```python
from build123d import *

# Parameters (mm, degrees)
BOSS_EXTRUDE1_DEPTH     = 40
SKETCH2_R               = 12.5
CUT_EXTRUDE1_DEPTH      = 4.4775
FILLET1_R               = 10
CUT_EXTRUDE2_DEPTH      = 131.2
CUT_EXTRUDE2_DEPTH_BACK = 14.2
SKETCH4_R               = 2.5
SKETCH6_W               = 68
SKETCH6_H               = 90
BOSS_EXTRUDE4_DEPTH     = 10
FILLET2_R               = 10
FILLET3_R               = 5
FILLET4_R               = 4
CUT_EXTRUDE3_START      = -2.2025
SKETCH7_R               = 3.9
CUT_EXTRUDE3_DEPTH      = 0.85
SKETCH8_R               = 3.25
CUT_EXTRUDE4_DEPTH      = 10
SKETCH9_R               = 4.025
CUT_EXTRUDE5_DEPTH      = 12
SKETCH10_W              = 20.05
SKETCH10_H              = 20.05
CUT_EXTRUDE6_DEPTH      = 4
CUT_EXTRUDE7_DEPTH      = 6
CUT_EXTRUDE9_DEPTH      = 2.5
CUT_EXTRUDE10_REACH     = 138.104
CUT_EXTRUDE10_START     = -2.5
SKETCH15_R              = 1.5
FILLET5_R               = 3


with BuildPart() as part:
    # Sketch1 → Boss-Extrude1 (new body)
    with BuildSketch(Plane.XY):
        Polygon((10, 0), (10, 43), (104, 43), (104, 0), (114, 0), (114, 53), (0, 53), (0, 0), align=None)
    extrude(amount=-BOSS_EXTRUDE1_DEPTH)

    # Sketch2 → Cut-Extrude1 (cut)
    with BuildSketch(Plane(origin=(10, 0, 0), x_dir=(0, 0, -1), z_dir=(1, 0, 0))):
        with Locations((20, 19.635146369)):
            Circle(SKETCH2_R)
    extrude(amount=-CUT_EXTRUDE1_DEPTH, mode=Mode.SUBTRACT)

    # Fillet1
    fillet1_edges = [part.edges().sort_by_distance(p)[0] for p in [
        (5, 0, 0),
        (109, 0, -40),
        (5, 0, -40),
        (109, 0, 0),
    ]]
    fillet(fillet1_edges, radius=FILLET1_R)

    # Sketch4 → Cut-Extrude2 (cut, two sides: drawn at the far end of the back side and taken through both)
    with BuildSketch(Plane(origin=(7.725, 0, 0), x_dir=(0, 0, -1), z_dir=(1, 0, 0)).offset(-CUT_EXTRUDE2_DEPTH_BACK)):
        with Locations(Location((20, 19.635146369, 0), (0, 0, 180))):
            Circle(SKETCH4_R)
    extrude(amount=CUT_EXTRUDE2_DEPTH + CUT_EXTRUDE2_DEPTH_BACK, mode=Mode.SUBTRACT)

    # Sketch6 → Boss-Extrude4 (add)
    with BuildSketch(Plane(origin=(0, 53, 0), x_dir=(1, 0, 0), z_dir=(0, 1, 0))):
        with Locations((57, 20)):
            Rectangle(SKETCH6_W, SKETCH6_H)
    extrude(amount=-BOSS_EXTRUDE4_DEPTH)

    # Fillet2
    fillet2_edges = [part.edges().sort_by_distance(p)[0] for p in [
        (23, 48, 0),
        (91, 48, 0),
        (91, 48, -40),
        (23, 48, -40),
    ]]
    fillet(fillet2_edges, radius=FILLET2_R)

    # Fillet3
    fillet3_edges = [part.edges().sort_by_distance(p)[0] for p in [
        (23, 48, 25),
        (91, 48, -65),
        (91, 48, 25),
        (23, 48, -65),
    ]]
    fillet(fillet3_edges, radius=FILLET3_R)

    # Fillet4
    fillet4_edges = [part.edges().sort_by_distance(p)[0] for p in [
        (0, 53, -20),
        (114, 53, -20),
    ]]
    fillet(fillet4_edges, radius=FILLET4_R)

    # Sketch7 → Cut-Extrude3 (cut)
    with BuildSketch(Plane(origin=(7.725, 0, 0), x_dir=(0, 0, -1), z_dir=(1, 0, 0)).offset(CUT_EXTRUDE3_START)):
        with Locations((20, 19.635146369)):
            Circle(SKETCH7_R)
    extrude(amount=-CUT_EXTRUDE3_DEPTH, mode=Mode.SUBTRACT)

    # Sketch8 → Cut-Extrude4 (cut)
    with BuildSketch(Plane(origin=(0, 53, 0), x_dir=(1, 0, 0), z_dir=(0, 1, 0))):
        with Locations(Location((57, 20, 0), (0, 0, 270))):
            Circle(SKETCH8_R)
    extrude(amount=-CUT_EXTRUDE4_DEPTH, mode=Mode.SUBTRACT)

    # Sketch9 → Cut-Extrude5 (cut)
    with BuildSketch(Plane(origin=(114, 0, 0), x_dir=(0, 0, -1), z_dir=(1, 0, 0))):
        with Locations(Location((20, 19.635146369, 0), (0, 0, 90))):
            Circle(SKETCH9_R)
    extrude(amount=-CUT_EXTRUDE5_DEPTH, mode=Mode.SUBTRACT)

    # Sketch10 → Cut-Extrude6 (cut)
    with BuildSketch(Plane(origin=(114, 0, 0), x_dir=(0, 0, -1), z_dir=(1, 0, 0))):
        with Locations((20, 19.635146369)):
            Rectangle(SKETCH10_W, SKETCH10_H)
    extrude(amount=-CUT_EXTRUDE6_DEPTH, mode=Mode.SUBTRACT)

    # Sketch14 → Cut-Extrude7 (cut)
    with BuildSketch(Plane(origin=(0, 53, 0), x_dir=(1, 0, 0), z_dir=(0, 1, 0))):
        Polygon((56.872881106, 25.694991584), (61.872881106, 22.808240238), (61.872881106, 17.034737546), (56.872881106, 14.1479862), (51.872881106, 17.034737546), (51.872881106, 22.808240238), align=None)
    extrude(amount=-CUT_EXTRUDE7_DEPTH, mode=Mode.SUBTRACT)

    # Sketch18 → Cut-Extrude9 (cut)
    with BuildSketch(Plane.ZY.offset(-104)):
        Polygon((-15.048857438, 28.91356654), (-11.910134999, 28.91356654), (-10.270487153, 26.081726401), (-11.891583597, 23.249886262), (-15.151000849, 23.249886262), (-16.733963505, 26.081726401), align=None)
        Polygon((-23.266036495, 26.081726401), (-24.951142562, 28.91356654), (-28.089865001, 28.91356654), (-29.729512847, 26.081726401), (-28.108416403, 23.249886262), (-24.848999151, 23.249886262), align=None)
        Polygon((-16.733963505, 13.188566337), (-15.048857438, 10.356726198), (-11.910134999, 10.356726198), (-10.270487153, 13.188566337), (-11.891583597, 16.020406476), (-15.151000849, 16.020406476), align=None)
        Polygon((-24.848999151, 16.020406476), (-23.266036495, 13.188566337), (-24.951142562, 10.356726198), (-28.089865001, 10.356726198), (-29.729512847, 13.188566337), (-28.108416403, 16.020406476), align=None)
    extrude(amount=-CUT_EXTRUDE9_DEPTH, mode=Mode.SUBTRACT)

    # Sketch15 → Cut-Extrude10 (cut, up to next)
    with BuildSketch(Plane.ZY.offset(-104).offset(CUT_EXTRUDE10_START), mode=Mode.PRIVATE) as cut_extrude10_sk1:
        with Locations(Location((-26.5, 26.135146369, 0), (0, 0, 270))):
            Circle(SKETCH15_R)
    cut_extrude10_tool1 = extrude(cut_extrude10_sk1.sketch, amount=-CUT_EXTRUDE10_REACH, mode=Mode.PRIVATE) & part.part
    # Sketch15 → Cut-Extrude10 (cut, up to next)
    with BuildSketch(Plane.ZY.offset(-104).offset(CUT_EXTRUDE10_START), mode=Mode.PRIVATE) as cut_extrude10_sk2:
        with Locations(Location((-13.5, 26.135146369, 0), (0, 0, 270))):
            Circle(SKETCH15_R)
    cut_extrude10_tool2 = extrude(cut_extrude10_sk2.sketch, amount=-CUT_EXTRUDE10_REACH, mode=Mode.PRIVATE) & part.part
    # Sketch15 → Cut-Extrude10 (cut, up to next)
    with BuildSketch(Plane.ZY.offset(-104).offset(CUT_EXTRUDE10_START), mode=Mode.PRIVATE) as cut_extrude10_sk3:
        with Locations(Location((-13.5, 13.135146369, 0), (0, 0, 270))):
            Circle(SKETCH15_R)
    cut_extrude10_tool3 = extrude(cut_extrude10_sk3.sketch, amount=-CUT_EXTRUDE10_REACH, mode=Mode.PRIVATE) & part.part
    # Sketch15 → Cut-Extrude10 (cut, up to next)
    with BuildSketch(Plane.ZY.offset(-104).offset(CUT_EXTRUDE10_START), mode=Mode.PRIVATE) as cut_extrude10_sk4:
        with Locations(Location((-26.5, 13.135146369, 0), (0, 0, 270))):
            Circle(SKETCH15_R)
    cut_extrude10_tool4 = extrude(cut_extrude10_sk4.sketch, amount=-CUT_EXTRUDE10_REACH, mode=Mode.PRIVATE) & part.part
    add(cut_extrude10_tool1.solids().sort_by_distance((106.5, 26.135146, -26.5))[0], mode=Mode.SUBTRACT)
    add(cut_extrude10_tool2.solids().sort_by_distance((106.5, 26.135146, -13.5))[0], mode=Mode.SUBTRACT)
    add(cut_extrude10_tool3.solids().sort_by_distance((106.5, 13.135146, -13.5))[0], mode=Mode.SUBTRACT)
    add(cut_extrude10_tool4.solids().sort_by_distance((106.5, 13.135146, -26.5))[0], mode=Mode.SUBTRACT)

    # Fillet5
    fillet5_edges = [part.edges().sort_by_distance(p)[0] for p in [
        (104, 43, -20),
        (10, 43, -20),
    ]]
    fillet(fillet5_edges, radius=FILLET5_R)


solid = part.part
```
Design review of the part built by this model. Coordinates are the model's own, in mm. A direction names the side the tool comes from. Round coordinates to 2 decimals unless told otherwise and drop trailing zeros. Write each loop counter-clockwise with the first axis right and the second up, starting at its lowest first coordinate (ties: lowest second). Pieces come first, ordered by that corner, then holes. Notation, with made-up numbers: (21.5, -8) -> (36.5, -8) arc R18 cw to (36.5, 27) -> close; hole circle Ø6 at (84, 68.5). An arc over 180 degrees is marked (long way). Answer in a Markdown table with one row per item.
Q1. Take a section at D-D, the plane x = 40. State the section outline as (y, z) points.
The answers:
| item | result |
|---|---|
| outline | (43, -65) -> (53, -65) -> (53, 25) -> (43, 25) -> close |
Q2. Take a section at B-B, the plane z = -36. State the section outline as (x, y) points.
The answers:
| item | result |
|---|---|
| outline | (0, 2) -> (10, 2) -> (10, 40) arc R3 cw to (13, 43) -> (101, 43) arc R3 cw to (104, 40) -> (104, 2) -> (114, 2) -> (114, 49) arc R4 ccw to (110, 53) -> (4, 53) arc R4 ccw to (0, 49) -> close |
Q3. To check wall thickness, follow L1, parallel to X at y = 30, z = -2; L2, parallel to Y at x = 5, z = -20; L3, parallel to Y at x = 8.5, z = -20. State the ranges of each line that lie inside material, in increasing order. Write a range as [from, to].
The answers:
| item | result |
|---|---|
| L1 | [0, 10], [104, 114] |
| L2 | [0, 15.74], [23.54, 53] |
| L3 | [0, 7.14], [32.14, 53] |
Q4. Draft analysis for pull direction Z (two halves, no side actions). For faces 1 (the face through (1.203, 51.859, -20.28)), 2 (the face through (24, 48, -63)), 3 (the face through (105, 23.25, -13)), state which applies: +Z half, -Z half, draft (parallel to the pull), parting line (faces both ways), or undercut.
The answers:
| item | result |
|---|---|
| face 1 | draft |
| face 2 | -Z half |
| face 3 | undercut |
Q5. For faces 4 (the face through (105.232, 24.646, -24.069)), 5 (the face through (91, 48, -55)), 6 (the face through (5, 32, -40)), 7 (the face through (112, 19, -9.975)), list the 3-axis set-ups (+Z, -Z, +X, -X, +Y, -Y) from which the entire face can be reached by the end or side of a thin tool; tool diameter is ignored.
The answers:
| item | result |
|---|---|
| face 4 | none |
| face 5 | -Z, +X, +Y, -Y |
| face 6 | -Z, -X, +Y, -Y |
| face 7 | +X |
Q6. Take a section at C-C, the plane z = -20. Count the separate pieces of the cut face and the enclosed holes in it, then the cut area to 3 significant figures.
The answers:
| item | result |
|---|---|
| separate pieces | 4 |
| enclosed holes | 0 |
| area | 1,640 mm² |
Q7. Clearance check with flat-ended pins moving along their axes: pin 1 Ø8.5 at (x, z) = (57, -20) entering from +Y; pin 2 Ø8 at (y, z) = (8.5, -3.5) entering from -X; pin 3 Ø10.5 at (x, y) = (110, 25.5) entering from -Z; pin 4 Ø1.5 at (x, z) = (93, -52) entering from -Y. State where each tip first meets the part, or that it passes through.
The answers:
| item | result |
|---|---|
| pin 1 | y = 47 |
| pin 2 | x = 0 |
| pin 3 | z = -40 |
| pin 4 | through |
Q8. Take a section at A-A, the plane y = 45. State the section outline as (x, z) points.
The answers:
| item | result |
|---|---|
| outline | (0, -40) -> (13, -40) arc R10 cw to (23, -50) -> (23, -60) arc R5 ccw to (28, -65) -> (86, -65) arc R5 ccw to (91, -60) -> (91, -50) arc R10 cw to (101, -40) -> (114, -40) -> (114, 0) -> (101, 0) arc R10 cw to (91, 10) -> (91, 20) arc R5 ccw to (86, 25) -> (28, 25) arc R5 ccw to (23, 20) -> (23, 10) arc R10 cw to (13, 0) -> (0, 0) -> close; hole circle Ø6.5 at (57, -20) |
